CAD build for the part. Positions are in the model's coordinates, mm. A direction names the side the tool comes from. Round coordinates to 2 decimals unless told otherwise and drop trailing zeros. Order: outer loops, then holes, each group sorted by start corner. A loop starts at its lowest first (then second) coordinate and runs counter-clockwise, first axis right, second up. Notation, with made-up numbers: M -33,19.25 L -2,19.25 A19 ccw -2,32.25 Z; hole C -26,37 d1. An arc over 180 degrees is marked long. Answer as a JSON object with one key per item and string values.
```python
from build123d import *

# Parameters (mm, degrees)
SKETCH_1_W          = 5
SKETCH_1_H          = 10
SKETCH_1_W_2        = 10
SKETCH_1_H_2        = 5
EXTRUDE_1_DEPTH     = 5
SKETCH_1_3_W        = 5
SKETCH_1_3_H        = 10
SKETCH_1_3_W_2      = 10
SKETCH_1_3_H_2      = 5
EXTRUDE_2_DEPTH     = 20
CUT_EXTRUDE_1_DEPTH = 20


with BuildPart() as part:
    # Sketch 1 → Extrude 1 (new body)
    with BuildSketch(Plane(origin=(0, 0, 0), x_dir=(1, 0, 0), z_dir=(0, 1, 0))):
        with Locations((-15, 5)):
            Rectangle(SKETCH_1_W, SKETCH_1_H)
        Polygon((-12.5, 0), (2.5, 0), (7.5, 5), (7.5, 10), (-12.5, 10), align=None)
        Polygon((7.5, 5), (2.5, 0), (-12.5, 0), (-17.5, 0), (-17.5, -10), (17.5, -10), (17.5, 5), align=None)
        with Locations((12.5, 7.5)):
            Rectangle(SKETCH_1_W_2, SKETCH_1_H_2)
    extrude(amount=EXTRUDE_1_DEPTH)

    # Sketch 1_3 → Extrude 2 (add)
    with BuildSketch(Plane(origin=(0, 0, 0), x_dir=(1, 0, 0), z_dir=(0, 1, 0))):
        with Locations((-15, 5)):
            Rectangle(SKETCH_1_3_W, SKETCH_1_3_H)
        Polygon((-12.5, 0), (2.5, 0), (7.5, 5), (7.5, 10), (-12.5, 10), align=None)
        with Locations((12.5, 7.5)):
            Rectangle(SKETCH_1_3_W_2, SKETCH_1_3_H_2)
    extrude(amount=EXTRUDE_2_DEPTH)

    # Sketch 2 → Cut-Extrude 1 (cut)
    with BuildSketch(Plane.XY):
        with BuildLine():
            Line((-12.5, 20), (-2.5, 20))
            ThreePointArc((-2.5, 20), (-7.5, 15), (-12.5, 20))
        make_face()
        Polygon((17.5, 5), (7.5, 20), (17.5, 20), align=None)
    extrude(amount=-CUT_EXTRUDE_1_DEPTH, mode=Mode.SUBTRACT)


solid = part.part
```
Item 1: Saw through at B-B on x = -13.5. List the corners of the cut face in (y, z).
Worked answers:
{"outline": "M 0,-10 L 20,-10 L 20,0 L 5,0 L 5,10 L 0,10 Z"}
Item 2: Wall check: line 1 along X through (y, z) = (16.5, -7); line 2 along Y through (x, z) = (9.5, 6.5); line 3 along Z through (x, y) = (9.5, 8.25). Give the ranges that are in metal, low to high. Write a range as [from, to].
Worked answers:
{"line 1": "x = [-17.5, -11.07], [-3.93, 9.83]", "line 2": "y = [0, 5]", "line 3": "z = [-10, -5]"}
Item 3: Saw through at C-C on y = 11. List the corners of the cut face in (x, z), and give its area (4 significant figures).
Worked answers:
{"outline": "M -17.5,-10 L 13.5,-10 L 13.5,-5 L 7.5,-5 L 2.5,0 L -17.5,0 Z", "area": "267.5 mm2"}
Item 4: 3-axis set-ups, long thin cutter, end or side, ignore diameter. For faces 1 (the flat face through (11, 11, -5)), 2 (the flat face through (-8, 11, 0)), 3 (the flat face through (-17.5, 8, -2)): which of +Z, -Z, +X, -X, +Y, -Y reach the whole face in a straight line?
Worked answers:
{"face 1": "+Z, +X, +Y", "face 2": "+Z, +X, -X, +Y", "face 3": "+Z, -Z, -X, +Y, -Y"}
Item 5: Saw through at D-D on z = -2. List the corners of the cut face in (x, y), and give its area (3 significant figures).
Worked answers:
{"outline": "M -17.5,0 L 17.5,0 L 17.5,5 L 4.5,5 L 4.5,20 L -2.5,20 A5 cw -12.5,20 L -17.5,20 Z", "area": "466 mm2"}
Item 6: Saw through at A-A on z = -8. List the corners of the cut face in (x, y), and give its area (3 significant figures).
Worked answers:
{"outline": "M -17.5,0 L 17.5,0 L 17.5,5 L 7.5,20 L -2.5,20 A5 cw -12.5,20 L -17.5,20 Z", "area": "586 mm2"}
Item 7: Drop flat-ended pins along their axis: pin 1 Ø1 at (y, z) = (6.5, -5) entering from +X; pin 2 Ø2 at (x, z) = (12, -3.5) entering from +Y; pin 3 Ø1 at (y, z) = (11, -2.5) entering from +X. Give the stop position or say it passes through.
Worked answers:
{"pin 1": "stops at x = 16.83", "pin 2": "stops at y = 5", "pin 3": "stops at x = 5.5"}
